from build123d import *

# Parameters (mm, degrees)
F1_DEPTH = 63.5
F2_DEPTH = 25.4
F3_DEPTH = 7.9375
F4_R     = 5.08


with BuildPart() as f1:
    # F0 (on Front) → F1 (new body, symmetric)
    with BuildSketch(Plane.XZ):
        Polygon((41.275, -9.525), (41.275, 9.525), (33.147, 9.525), (-41.275, 9.525), (-41.275, -9.525), align=None)
    extrude(amount=F1_DEPTH, both=True)

    # F0 (on Front) → F2 (join, symmetric)
    with BuildSketch(Plane.XZ):
        with BuildLine():
            Line((33.147, 9.525), (41.275, 9.525))
            Line((41.275, 9.525), (41.275, 39.270175))
            ThreePointArc((41.275, 39.270175), (45.92468, 50.495495), (57.15, 55.145175))
            Line((57.15, 55.145175), (83.04214, 55.145175))
            Line((83.04214, 55.145175), (83.04214, 63.273175))
            Line((83.04214, 63.273175), (57.15, 63.273175))
            ThreePointArc((57.15, 63.273175), (40.177316, 56.242859), (33.147, 39.270175))
            Line((33.147, 39.270175), (33.147, 9.525))
        make_face()
        Polygon((133.84214, 74.787841), (83.04214, 74.787841), (83.04214, 63.273175), (83.04214, 55.145175), (83.04214, 46.212841), (133.84214, 46.212841), align=None)
    extrude(amount=F2_DEPTH, both=True)

    # F0 (on Front) → F3 (join, symmetric)
    with BuildSketch(Plane.XZ):
        with BuildLine():
            Line((-41.275, 9.525), (33.147, 9.525))
            Line((33.147, 9.525), (33.147, 39.270175))
            ThreePointArc((33.147, 39.270175), (40.177316, 56.242859), (57.15, 63.273175))
            Line((57.15, 63.273175), (83.04214, 63.273175))
            Line((83.04214, 63.273175), (83.04214, 74.787841))
            add(Edge.make_bspline(
                [(-41.275, 9.525), (-10.652266, 69.008738), (42.873295, 67.373856), (83.04214, 74.787841)],
                knots=[0, 0, 0, 0, 140.406516, 140.406516, 140.406516, 140.406516], degree=3))
        make_face()
    extrude(amount=F3_DEPTH, both=True)

    # F4
    f4_edges = [f1.edges().sort_by_distance(p)[0] for p in [
        (-41.275, -63.5, 0),
        (41.275, -63.5, 0),
        (41.275, 63.5, 0),
        (-41.275, 63.5, 0),
    ]]
    fillet(f4_edges, radius=F4_R)


solid = f1.part
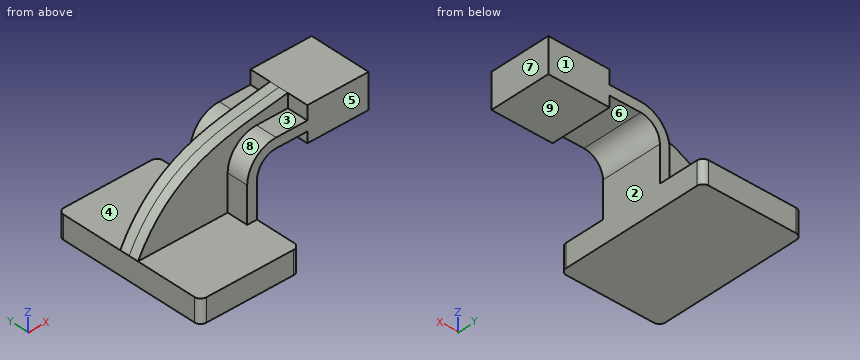
Input: part model. Units: mm. Frame: model coordinates. Face numbers are marked on the shaded views. A direction names the side the tool comes from. Coordinates: 2 decimals unless noted, no trailing zeros. Loops run counter-clockwise (first coordinate to the right, second up) from the corner with the lowest first, then second, coordinate; pieces in that order, holes last.
Q1. Cut plane A-A (z = -0.5). Output: boundary loops of the cut face in (x, y) (3 decimals), then the cut area to 3 significant figures.
Q2. Draft query along X for the marked faces 6, 7, 8 and 9. Return one class per face: +X half, -X half, draft (parallel to the pull), parting line (faces both ways), or undercut.
Q3. Cut plane B-B (x = 103.5). Output: boundary loops of the cut face in (y, z).
Q4. Contact query for flat-ended pins moving along their axis: pin 1 (14 mm diameter, centred on y = -14.5, z = 31, fed in from -X); pin 2 (2 mm diameter, centred on x = -0.5, y = -44.5, fed in from +Z) (3 decimals); pin 3 (7 mm diameter, centred on y = -6, z = 51, fed in from -X). Output: stop coordinate, or through.
Q5. Material intervals for line 1 (Z direction, x = 111, y = -17); line 2 (X direction, y = 18.5, z = 67); line 3 (Z direction, x = -19.5, y = -36) (3 decimals), sorted ascending.
Q6. Set-up query: the marked faces 1, 2, 3, 4 and 5. Return all of +Z, -Z, +X, -X, +Y, -Y with unobstructed straight access to the full face (end or side cutting, diameter ignored); none if empty.
Q7. Cut plane C-C (y = -27.5). Output: boundary loops of the cut face in (x, z) (3 decimals), then the cut area to 3 significant figures.
Working result:
1. outline: (-41.275, -58.42) arc R5.08 ccw to (-36.195, -63.5) - (36.195, -63.5) arc R5.08 ccw to (41.275, -58.42) - (41.275, 58.42) arc R5.08 ccw to (36.195, 63.5) - (-36.195, 63.5) arc R5.08 ccw to (-41.275, 58.42) - close
1. area: 10,500 mm2
2. face 6: undercut
2. face 7: +X half
2. face 8: -X half
2. face 9: draft
3. outline: (-25.4, 46.21) - (25.4, 46.21) - (25.4, 74.79) - (-25.4, 74.79) - close
4. pin 1: stops at x = -29.21
4. pin 2: stops at z = 9.525
4. pin 3: stops at x = -9.83
5. line 1: z = 46.21 to 74.79
5. line 2: x = 83.04 to 133.84
5. line 3: z = -9.525 to 9.525
6. face 1: +Z, +X, -X, +Y
6. face 2: -Z, +X, +Y, -Y
6. face 3: +Z, -X, -Y
6. face 4: +Z, -X, +Y
6. face 5: +Z, +X, -X, -Y
7. outline: (-41.275, -9.525) - (41.275, -9.525) - (41.275, 9.525) - (-41.275, 9.525) - close
7. area: 1,570 mm2
